Can you work these out from the model? Positions are in its coordinate system, mm. Face numbers are marked on the shaded views. A direction names the side the tool comes from. Give positions to 0.01 mm unless a question says otherwise; leave off trailing zeros. Order: outer loops, then holes, each group sorted by start corner. A loop starts at its lowest first (then second) coordinate and runs counter-clockwise, first axis right, second up. Notation, with made-up numbers: (77.5, -25) - (121.5, -25) arc R20 ccw to (121.5, 12) - close; hole circle Ø8 at (-27.75, 56.25). An arc over 180 degrees is marked (long way). Answer as a JSON object with one key per item and string values.
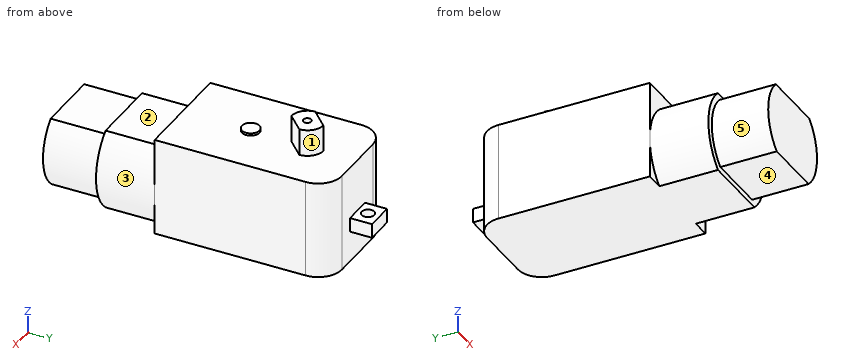
Autodesk Inventor part; units mm, degrees
ref_plane "YZ Plane" through (0, 0, 0) normal (1, 0, 0) x (0, 1, 0)
ref_plane "XZ Plane" through (0, 0, 0) normal (0, 1, 0) x (-1, 0, 0)
ref_plane "XY Plane" through (0, 0, 0) normal (0, 0, 1) x (1, 0, 0)
sketch "Sketch1" plane through (0, 0, 0) normal (0, 0, 1) x (1, 0, 0)
  line L0 (-6.2484, 18.5674) -> (6.2484, 18.5674)
  line L1 (11.3284, 13.4874) -> (11.3284, -18.5674)
  line L2 (11.3284, -18.5674) -> (-11.3284, -18.5674)
  line L3 (-11.3284, -18.5674) -> (-11.3284, 13.4874)
  line L4 (-11.3284, 18.5674) -> (11.3284, -18.5674) construction
  line L5 (11.3284, 18.5674) -> (-11.3284, -18.5674) construction
  arc A0 (-6.2484, 18.5674) -> (-11.3284, 13.4874) centre (-6.2484, 13.4874) ccw
  arc A1 (11.3284, 13.4874) -> (6.2484, 18.5674) centre (6.2484, 13.4874) ccw
  point P0 (0, 0)
  dimension "d1" = 37.1348
  dimension "d2" = 5.08
  dimension "d45" = 22.6568
extrude "Extrusion1" add sketch "Sketch1" along normal blind 20.828
sketch "Sketch2" plane through (0, 0, 20.828) normal (0, 0, 1) x (1, 0, 0)
  line L0 (-3.4946, 7.7761) -> (0.1481, 11.4046)
  line L1 (3.4167, 7.9922) -> (-0.097, 4.4922)
  line L2 (6.2484, 18.5674) -> (-6.2484, 18.5674)
  arc A0 (3.4167, 7.9922) -> (0.1481, 11.4046) centre (-0.0127, 7.9789) ccw
  arc A1 (-3.4946, 7.7761) -> (-0.097, 4.4922) centre (-0.0127, 7.9789) ccw
  point P0 (0, 0)
  dimension "d9" = 7.1628
  dimension "d11" = 4.7244
extrude "Extrusion2" add sketch "Sketch2" along normal blind 5.6896
sketch "Sketch3" plane through (0, 0, 26.5176) normal (0, 0, 1) x (1, 0, 0)
  circle A0 centre (0, 7.9106) radius 0.8509
  point P0 (0, 0)
  dimension "d14" = 1.7018
extrude "Extrusion3" cut sketch "Sketch3" against normal blind 5.5372
sketch "Sketch4" plane through (-6.2484, 18.5674, 0) normal (0, 1, 0) x (1, 0, 0)
  line L0 (3.2004, -6.604) -> (9.2964, -6.604)
  line L1 (9.2964, -6.604) -> (9.2964, -9.6266)
  line L2 (9.2964, -9.6266) -> (3.2004, -9.6266)
  line L3 (3.2004, -9.6266) -> (3.2004, -6.604)
  line L4 (3.2004, -6.604) -> (9.2964, -9.6266) construction
  line L5 (9.2964, -6.604) -> (3.2004, -9.6266) construction
  line L6 (12.4968, 0) -> (0, 0)
  point P0 (6.2484, 0)
  point P1 (6.2484, -8.1153)
  point P2 (6.2484, -8.1153)
  point P3 (6.2484, 0)
  dimension "d17" = 6.096
  dimension "d18" = 3.0226
  dimension "d19" = 6.604
extrude "Extrusion4" add sketch "Sketch4" along normal blind 4.6736
sketch "Sketch5" plane through (-3.048, 18.5674, 9.6266) normal (0, 0, 1) x (1, 0, 0)
  circle A0 centre (3.048, 2.2411) radius 1.3462
  point P0 (3.048, -18.5674)
  dimension "d22" = 2.6924
extrude "Extrusion5" cut sketch "Sketch5" against normal blind 4.6736 and the other way blind 2.3368
sketch "Sketch6" plane through (0, 0, 20.828) normal (0, 0, 1) x (1, 0, 0)
  circle A0 centre (0, -4.0871) radius 1.8669
  line L0 (-0.097, 4.4922) -> (3.4167, 7.9922)
  point P0 (0, 0)
  dimension "d27" = 3.7338
  dimension "d28" = 6.1468
extrude "Extrusion6" add sketch "Sketch6" along normal blind 0.508
sketch "Sketch8" plane through (-11.3284, -18.5674, 0) normal (0, -1, 0) x (1, 0, 0)
  line L0 (0, 0) -> (22.6568, 0)
  line L1 (3.8934, 17.0942) -> (18.7634, 17.0942)
  line L2 (22.6568, 17.0942) -> (22.6568, 0)
  line L3 (22.6568, 0) -> (0, 0)
  line L4 (0, 0) -> (0, 17.0942)
  line L5 (0, 20.828) -> (22.6568, 20.828)
  line L6 (22.6568, 0) -> (22.6568, 20.828)
  arc A0 (18.7634, 0) -> (18.7634, 17.0942) centre (11.3284, 8.5471) ccw
  arc A1 (3.8934, 17.0942) -> (3.8934, 0) centre (11.3284, 8.5471) ccw
  point P0 (11.3284, 0)
  point P1 (11.3284, 8.5471)
  point P2 (11.3284, 20.828)
extrude "Extrusion8" add sketch "Sketch8" along normal blind 12.446 contours A1 L1 A0 L0
sketch "Sketch9" plane through (-11.3284, -31.0134, 0) normal (0, -1, 0) x (1, 0, 0)
  line L0 (4.4951, 15.9258) -> (18.1617, 15.9258)
  line L1 (17.8198, 1.1684) -> (4.837, 1.1684)
  arc A0 (4.4951, 15.9258) -> (4.837, 1.1684) centre (11.3284, 8.7014) ccw
  arc A1 (17.8198, 1.1684) -> (18.1617, 15.9258) centre (11.3284, 8.7014) ccw
  line L2 (18.7634, 17.0942) -> (3.8934, 17.0942)
  line L3 (3.8934, 0) -> (18.7634, 0)
  point P0 (11.3284, 0)
  point P1 (11.3284, 8.7014)
  point P2 (11.3284, 8.7014)
  point P3 (11.3284, 8.7014)
  dimension "d53" = 1.1684
  dimension "d54" = 1.1684
extrude "Extrusion9" add sketch "Sketch9" along normal blind 11.9634
properties part number "Motor"
Q1. If we section it at C-C, the plane y = -5: Please give me the cut outline in (x, z), then the cut area to 3 significant figures.
Recorded:
{"outline": "(-11.33, 0) - (11.33, 0) - (11.33, 20.83) - (1.63, 20.83) - (1.63, 21.34) - (-1.63, 21.34) - (-1.63, 20.83) - (-11.33, 20.83) - close", "area": "474 mm^2"}
Q2. I'm going to push flat-ended pins straight in: pin 1 Ø3.5 at (x, y) = (-2.5, -36) entering from +Z; pin 2 Ø3.5 at (y, z) = (20.5, 8.5) entering from +X; pin 3 Ø1.5 at (x, z) = (-8.5, 21) entering from +Y. Where does each tip first touch, or does it pass through?
Recorded:
{"pin 1": "stops at z = 15.93", "pin 2": "stops at x = 3.05", "pin 3": "stops at y = 18.33"}
Q3. If we section it at D-D, the plane z = 25: Please give me the cut outline in (x, y), then the cut area to 3 significant figures.
Recorded:
{"outline": "(-3.49, 7.78) arc R3.49 ccw to (-0.1, 4.49) - (3.42, 7.99) arc R3.43 ccw to (0.15, 11.4) - close; hole circle Ø1.7 at (0, 7.91)", "area": "27.6 mm^2"}
Q4. If we section it at B-B, the plane x = -9.25: Please give me the cut outline in (y, z).
Recorded:
{"outline": "(-42.98, 5.05) - (-31.01, 5.05) - (-31.01, 2.01) - (-18.57, 2.01) - (-18.57, 0) - (17.59, 0) - (17.59, 20.83) - (-18.57, 20.83) - (-18.57, 15.09) - (-31.01, 15.09) - (-31.01, 12.35) - (-42.98, 12.35) - close"}
Q5. I need wall thicknesses on L1, parallel to Y at x = 0, z = 8.35; L2, parallel to Z at x = -3, y = -15; L3, parallel to Y at x = -4.75, z = 4.75. Which ranges of each line are inside material? Lowest first, please.
Recorded:
{"L1": "y = -42.98 to 19.46, 22.15 to 23.24", "L2": "z = 0 to 20.83", "L3": "y = -42.98 to 18.57"}
Q6. If we section it at A-A, the plane z = 5.5: Please give me the cut outline in (x, y), then the cut area to 3 significant figures.
Recorded:
{"outline": "(-11.33, -18.57) - (-10.91, -18.57) - (-10.91, -31.01) - (-9.41, -31.01) - (-9.41, -42.98) - (9.41, -42.98) - (9.41, -31.01) - (10.91, -31.01) - (10.91, -18.57) - (11.33, -18.57) - (11.33, 13.49) arc R5.08 ccw to (6.25, 18.57) - (-6.25, 18.57) arc R5.08 ccw to (-11.33, 13.49) - close", "area": "1,330 mm^2"}
Q7. Which directions (+Z, -Z, +X, -X, +Y, -Y) give clear straight access to the entire face, cutting with the end or side of a thin tool? Please do the marked faces 1, 2, 3, 4 and 5.
Recorded:
{"face 1": "+Z, +X, +Y", "face 2": "+Z, +X, -X, -Y", "face 3": "+X, -Y", "face 4": "-Z, +X, -X, -Y", "face 5": "-X, -Y"}
